Check sheet for the modelled part. Datum: model origin and axes. Units: mm. Round coordinates to 2 decimals unless told otherwise and drop trailing zeros. Order: outer loops, then holes, each group sorted by start corner. A loop starts at its lowest first (then second) coordinate and runs counter-clockwise, first axis right, second up.
```python
from build123d import *

# Parameters (mm, degrees)
SKETCH_1_W                 = 160
SKETCH_1_H                 = 100
EXTRUDE_1_DEPTH            = 1.6
FILLET_1_R                 = 2
HOLE_WIZARD_M3_1_OUTLINE_R = 1.6
HOLE_WIZARD_M3_1_DEPTH     = 1.6


# Read off the part's stored shape, not the designer's step: M3 すきま穴1
with BuildPart() as part:
    # ｽｹｯﾁ1 → ﾎﾞｽ - 押し出し1 (new body)
    with BuildSketch(Plane.XY):
        Rectangle(SKETCH_1_W, SKETCH_1_H)
    extrude(amount=EXTRUDE_1_DEPTH)

    # ﾌｨﾚｯﾄ1
    fillet_1_edges = [part.edges().sort_by_distance(p)[0] for p in [
        (-80, 50, 0.8),
        (80, 50, 0.8),
        (80, -50, 0.8),
        (-80, -50, 0.8),
    ]]
    fillet(fillet_1_edges, radius=FILLET_1_R)

    # M3 すきま穴1 outline → M3 すきま穴1 (cut)
    with BuildSketch(Plane.XY):
        with Locations((75, -45)):
            Circle(HOLE_WIZARD_M3_1_OUTLINE_R)
        with Locations((-75, 45)):
            Circle(HOLE_WIZARD_M3_1_OUTLINE_R)
        with Locations((-75, -45)):
            Circle(HOLE_WIZARD_M3_1_OUTLINE_R)
        with Locations((75, 45)):
            Circle(HOLE_WIZARD_M3_1_OUTLINE_R)
    extrude(amount=HOLE_WIZARD_M3_1_DEPTH, mode=Mode.SUBTRACT)


solid = part.part
```
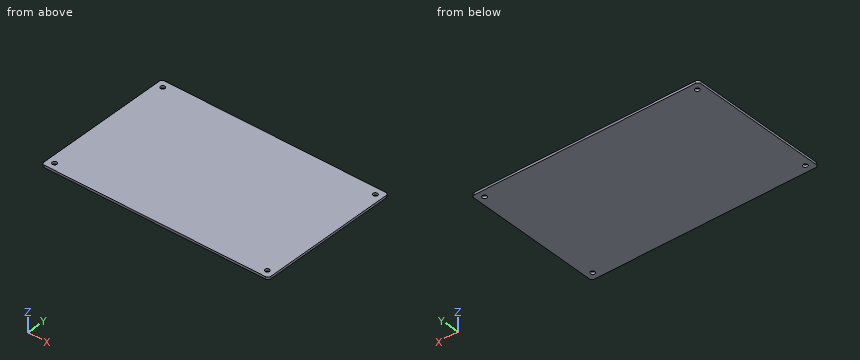
Item 1: Sectioned sample at A-A (x = -75). Record the cut outline in (y, z), and give its area (3 significant figures).
Answer:
outline: (-50, 0) - (-46.6, 0) - (-46.6, 1.6) - (-50, 1.6) - close; (-43.4, 0) - (43.4, 0) - (43.4, 1.6) - (-43.4, 1.6) - close; (46.6, 0) - (50, 0) - (50, 1.6) - (46.6, 1.6) - close
area: 150 mm2
Item 2: Sectioned sample at B-B (y = 45). Record the cut outline in (x, z).
Answer:
outline: (-80, 0) - (-76.6, 0) - (-76.6, 1.6) - (-80, 1.6) - close; (-73.4, 0) - (73.4, 0) - (73.4, 1.6) - (-73.4, 1.6) - close; (76.6, 0) - (80, 0) - (80, 1.6) - (76.6, 1.6) - close
Item 3: Scan line: line 1 along Y through (x, z) = (75, 0.7). Record every from-to range of solid material in increasing order.
Answer:
line 1: y = -50 to -46.6, -43.4 to 43.4, 46.6 to 50
Item 4: Go/stop test with a flat-tipped pin: P1, Ø1.9, axis at x = 75, y = -45, coming from the +Z side. Record where the tip stops, or that it passes through.
Answer:
P1: passes through
